Here's how the part is built. I have some questions about the finished solid (model axes, mm). Face numbers are marked on the shaded views. Round coordinates to 2 decimals unless told otherwise and drop trailing zeros. Write each loop counter-clockwise with the first axis right and the second up, starting at its lowest first coordinate (ties: lowest second). Pieces come first, ordered by that corner, then holes. Notation, with made-up numbers: M -16,70.25 L -6,70.25 A19 cw -6,90.25 Z; hole C -9.75,78 d1. An arc over 180 degrees is marked long. Use a Markdown table: item, result. Add a question column.
Autodesk Inventor part; units mm, degrees
ref_plane "YZ Plane" through (0, 0, 0) normal (1, 0, 0) x (0, 1, 0)
ref_plane "XZ Plane" through (0, 0, 0) normal (0, 1, 0) x (-1, 0, 0)
ref_plane "XY Plane" through (0, 0, 0) normal (0, 0, 1) x (1, 0, 0)
sketch "Sketch1" plane through (0, 0, 0) normal (0, 1, 0) x (-1, 0, 0)
  line L0 (22, 22) -> (-22, 22)
  line L1 (-22, 22) -> (-22, -22)
  line L2 (-22, -22) -> (22, -22)
  line L3 (22, -22) -> (22, 22)
  line L4 (22, 22) -> (-22, -22) construction
  line L5 (-22, 22) -> (22, -22) construction
  point P0 (0, 0)
  dimension "d0" = 44
  dimension "d1" = 44
extrude "Extrusion1" add sketch "Sketch1" along normal blind 6
sketch "Sketch2" plane through (0, 6, 0) normal (0, 1, 0) x (1, 0, 0)
  line L0 (-20.3, -20.3) -> (20.3, -20.3)
  line L1 (20.3, -20.3) -> (20.3, 20.3)
  line L2 (20.3, 20.3) -> (-20.3, 20.3)
  line L3 (-20.3, 20.3) -> (-20.3, -20.3)
  line L4 (-20.3, -20.3) -> (20.3, 20.3) construction
  line L5 (20.3, -20.3) -> (-20.3, 20.3) construction
  point P0 (0, 0)
  dimension "d4" = 40.6
  dimension "d5" = 40.6
extrude "Extrusion2" cut sketch "Sketch2" against normal blind 1.6
sketch "Sketch3" plane through (0, 4.4, 0) normal (0, 1, 0) x (1, 0, 0)
  line L0 (-19.3, -19.3) -> (19.3, -19.3)
  line L1 (19.3, -19.3) -> (19.3, 19.3)
  line L2 (19.3, 19.3) -> (-19.3, 19.3)
  line L3 (-19.3, 19.3) -> (-19.3, -19.3)
  line L4 (-19.3, -19.3) -> (19.3, 19.3) construction
  line L5 (19.3, -19.3) -> (-19.3, 19.3) construction
  point P0 (0, 0)
  dimension "d8" = 38.6
  dimension "d9" = 38.6
extrude "Extrusion3" cut sketch "Sketch3" against normal blind 3.4
sketch "Sketch4" plane through (0, 1, 0) normal (0, 1, 0) x (1, 0, 0)
  circle A0 centre (-15.3, 15.3) radius 3
  circle A1 centre (15.3, -15.3) radius 3
  line L0 (-20.3, 20.3) -> (20.3, 20.3)
  line L1 (-20.3, -20.3) -> (-20.3, 20.3)
  line L2 (20.3, 20.3) -> (20.3, -20.3)
  line L3 (20.3, -20.3) -> (-20.3, -20.3)
  point P0 (0, 0)
  dimension "d12" = 5
  dimension "d13" = 5
  dimension "d14" = 6
  dimension "d15" = 5
  dimension "d16" = 5
  dimension "d17" = 6
extrude "Extrusion4" add sketch "Sketch4" along normal blind 3.4 contours A0 | A1
sketch "Sketch5" plane through (-15.3, 4.4, -15.3) normal (0, 1, 0) x (1, 0, 0)
  circle A0 centre (0, 0) radius 1
  circle A1 centre (30.6, -30.6) radius 3
  circle A2 centre (30.6, -30.6) radius 1
  point P0 (15.3, -15.3)
  dimension "d20" = 2
  dimension "d21" = 2
extrude "Extrusion5" cut sketch "Sketch5" against normal blind 3.4 contours A0 | A2
fillet "Fillet1" radius 2 4 edges at (-22, 3, -22) (22, 3, -22) (22, 3, 22) (-22, 3, 22)
properties part number "elec_detect_bucket"
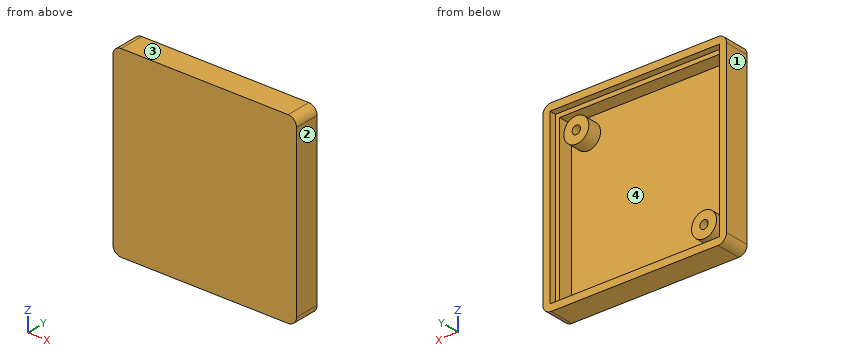
Item 1: Imagine slicing it at A-A on x = 15.3. List the corners of the cut face in (y, z) for me.
Item 2: For pin 1 Ø1.5 at (x, z) = (-9, 9.5) entering from +Y; pin 2 Ø1.8 at (x, z) = (-16.5, -16.5) entering from +Y, each with a flat end and sliding along its axis, tell me the tip position at first contact or that it passes through.
Item 3: I need wall thicknesses on probe 1 along Z at (x, y) = (15.3, 3.45); probe 2 along Z at (x, y) = (-15.3, 3.05). Which ranges of each line are inside material? Lowest first, please. Write a range as from..to.
Item 4: If we mould it in two halves opening along X, with no side actions, what happens to the marked faces 1, 2, 3 and 4? For each: +X half, -X half, draft (parallel to the pull), parting line (faces both ways), or undercut.
Item 5: Imagine slicing it at D-D on x = -4.5. List the corners of the cut face in (y, z) for me.
Item 6: Imagine slicing it at B-B on y = 5.1. List the corners of the cut face in (x, z) for me.
Item 7: Imagine slicing it at C-C on z = -15.3. List the corners of the cut face in (x, y) for me.
The answers:
| question | item | result |
|---|---|---|
| 1 | outline | M 0,-22 L 6,-22 L 6,-20.3 L 4.4,-20.3 L 4.4,-19.3 L 1,-19.3 L 1,12.3 L 4.4,12.3 L 4.4,14.3 L 1,14.3 L 1,16.3 L 4.4,16.3 L 4.4,18.3 L 1,18.3 L 1,19.3 L 4.4,19.3 L 4.4,20.3 L 6,20.3 L 6,22 L 0,22 Z |
| 2 | pin 1 | y = 1 |
| 2 | pin 2 | y = 4.4 |
| 3 | probe 1 | -22..-19.3, 12.3..14.3, 16.3..18.3, 19.3..22 |
| 3 | probe 2 | -22..-19.3, -18.3..-16.3, -14.3..-12.3, 19.3..22 |
| 4 | face 1 | -X half |
| 4 | face 2 | +X half |
| 4 | face 3 | draft |
| 4 | face 4 | undercut |
| 5 | outline | M 0,-22 L 6,-22 L 6,-20.3 L 4.4,-20.3 L 4.4,-19.3 L 1,-19.3 L 1,19.3 L 4.4,19.3 L 4.4,20.3 L 6,20.3 L 6,22 L 0,22 Z |
| 6 | outline | M -22,-20 A2 ccw -20,-22 L 20,-22 A2 ccw 22,-20 L 22,20 A2 ccw 20,22 L -20,22 A2 ccw -22,20 Z; hole M -20.3,-20.3 L 20.3,-20.3 L 20.3,20.3 L -20.3,20.3 Z |
| 7 | outline | M -22,0 L 22,0 L 22,6 L 20.3,6 L 20.3,4.4 L 19.3,4.4 L 19.3,1 L -12.3,1 L -12.3,4.4 L -14.3,4.4 L -14.3,1 L -16.3,1 L -16.3,4.4 L -18.3,4.4 L -18.3,1 L -19.3,1 L -19.3,4.4 L -20.3,4.4 L -20.3,6 L -22,6 Z |
